The model under review builds one solid part; all positions refer to its coordinate system, in mm. A direction names the side the tool comes from. Coordinates: 2 decimals unless noted, no trailing zeros. Loops run counter-clockwise (first coordinate to the right, second up) from the corner with the lowest first, then second, coordinate; pieces in that order, holes last. Notation, with made-up numbers: M 41.5,30 L 86.5,30 A10 cw 86.5,49 Z; hole C 0.25,69.25 d6. An arc over 180 degrees is marked long. Use CSV: the item, a comma, the result in double quotes. Start each with the question number.
1. Add section C-C, the plane x = 14.5. Write out the cut boundary in (y, z), then the cut area to 3 significant figures.
2. Add section A-A, the plane z = 12. Write out the cut boundary in (x, y), then the cut area to 3 significant figures.
3. Add section D-D, the plane y = 2. Write out the cut boundary in (x, z).
4. Clearance check with flat-ended pins moving along their axes: P1, Ø1, axis at x = 16, y = 3.5, coming from the +Z side; P2, Ø12, axis at x = 10.5, y = 12.5, coming from the +Z side; P3, Ø2.5, axis at x = 10.5, z = 7.5, coming from the -Y side. State where each tip first meets the part, or that it passes through.
5. Tool access review of faces 1 (the flat face through (20, 12.9, 3.7)), 2 (the flat face through (10, 16.902, 10)): name each direction out of +Z, -Z, +X, -X, +Y, -Y from which nothing blocks a thin tool from reaching the whole face with its end or side.
6. For L1, parallel to Y at x = 13.5, z = 9.75; L2, parallel to Z at x = 8, y = 20; L3, parallel to Z at x = 10, y = 16.75, list the stretches that pass through material, from the lowest coordinate up.
7. Draft analysis for pull direction Y (two halves, no side actions). For faces 3 (the flat face through (16, 19, 4.075)), 4 (the flat face through (10, 0, 10)), 5 (the flat face through (10, 12, 0)), state which applies: +Y half, -Y half, draft (parallel to the pull), parting line (faces both ways), or undercut.
8. Add section B-B, the plane x = 10. Write out the cut boundary in (y, z), then the cut area to 3 significant figures.
from build123d import *

# Parameters (mm, degrees)
BOSS_EXTRUDE2_DEPTH     = 20
CUT_EXTRUDE1_DEPTH      = 35.858058648
CUT_EXTRUDE1_DEPTH_BACK = 35.858058648
SKETCH3_R               = 2.962169801


with BuildPart() as part:
    # Sketch2 → Boss-Extrude2 (new body)
    with BuildSketch(Plane(origin=(0, 0, 0), x_dir=(0, 0, -1), z_dir=(1, 0, 0))):
        Polygon((0, 0), (0, 25.347810212), (-13.136695555, 25.347810212), (-13.136695555, 21.488272358), (-4.075171897, 21.488272358), (-4.075171897, 16.901575198), (-13.136695555, 16.901575198), (-13.136695555, 13.76919665), (-4.075171897, 13.76919665), (-4.075171897, 9.350305483), (-13.136695555, 9.350305483), (-13.136695555, 6.050120941), (-4.075171897, 6.050120941), (-4.075171897, 2.694001068), (-13.136695555, 2.694001068), (-13.136695555, 0), align=None)
    extrude(amount=BOSS_EXTRUDE2_DEPTH)

    # Sketch3 → Cut-Extrude1 (cut, two sides: drawn at the far end of the back side and taken through both)
    with BuildSketch(Plane(origin=(0, 25.347810212, 0), x_dir=(1, 0, 0), z_dir=(0, 1, 0)).offset(-CUT_EXTRUDE1_DEPTH_BACK)):
        with Locations(Location((10, -6.568347778, 0), (0, 0, 270))):
            Circle(SKETCH3_R)
    extrude(amount=CUT_EXTRUDE1_DEPTH + CUT_EXTRUDE1_DEPTH_BACK, mode=Mode.SUBTRACT)


solid = part.part
Computed:
1,outline,"M 0,0 L 25.35,0 L 25.35,13.14 L 21.49,13.14 L 21.49,4.08 L 16.9,4.08 L 16.9,13.14 L 13.77,13.14 L 13.77,4.08 L 9.35,4.08 L 9.35,13.14 L 6.05,13.14 L 6.05,4.08 L 2.69,4.08 L 2.69,13.14 L 0,13.14 Z"
1,area,"221 mm^2"
2,outline,"M 0,0 L 20,0 L 20,2.69 L 0,2.69 Z; M 0,6.05 L 20,6.05 L 20,9.35 L 0,9.35 Z; M 0,13.77 L 20,13.77 L 20,16.9 L 0,16.9 Z; M 0,21.49 L 20,21.49 L 20,25.35 L 0,25.35 Z"
2,area,"260 mm^2"
3,outline,"M 0,0 L 20,0 L 20,13.14 L 0,13.14 Z; hole C 10,6.57 d5.92"
4,P1,"stops at z = 4.08"
4,P2,"stops at z = 13.14"
4,P3,"passes through"
5,face 1,"+Z, -Z, +X, +Y, -Y"
5,face 2,"+Z, +X, -X"
6,L1,"y = 0 to 2.69, 6.05 to 9.35, 13.77 to 16.9, 21.49 to 25.35"
6,L2,"z = 0 to 4.08"
6,L3,"z = 0 to 3.61, 9.53 to 13.14"
7,face 3,"undercut"
7,face 4,"-Y half"
7,face 5,"draft"
8,outline,"M 0,0 L 25.35,0 L 25.35,3.61 L 0,3.61 Z; M 0,9.53 L 2.69,9.53 L 2.69,13.14 L 0,13.14 Z; M 6.05,9.53 L 9.35,9.53 L 9.35,13.14 L 6.05,13.14 Z; M 13.77,9.53 L 16.9,9.53 L 16.9,13.14 L 13.77,13.14 Z; M 21.49,9.53 L 25.35,9.53 L 25.35,13.14 L 21.49,13.14 Z"
8,area,"138 mm^2"
